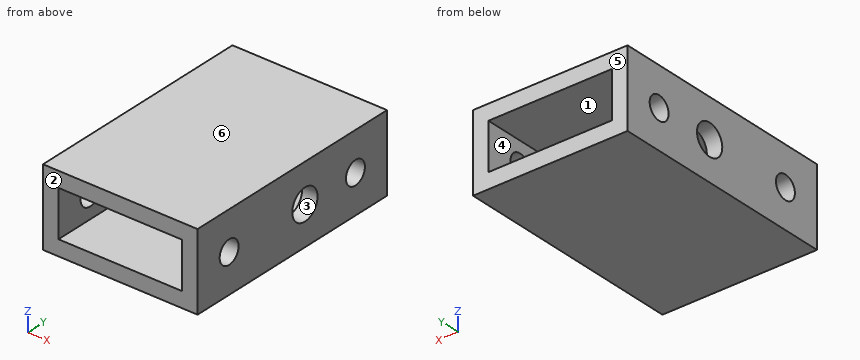
```python
from build123d import *

# Parameters (mm, degrees)
SKETCH_1_W          = 20
SKETCH_1_H          = 10
SKETCH_1_W_2        = 16
SKETCH_1_H_2        = 6
EXTRUDE_1_DEPTH     = 15
SKETCH_2_R          = 2
SKETCH_2_R_2        = 1.5
CUT_EXTRUDE_1_DEPTH = 26.495097568


with BuildPart() as part:
    # 草图1 → 凸台-拉伸1 (new, symmetric)
    with BuildSketch(Plane(origin=(0, 0, 0), x_dir=(1, 0, 0), z_dir=(0, 1, 0))):
        Rectangle(SKETCH_1_W, SKETCH_1_H)
        Rectangle(SKETCH_1_W_2, SKETCH_1_H_2, mode=Mode.SUBTRACT)
    extrude(amount=EXTRUDE_1_DEPTH, both=True)

    # 草图2 → 切除-拉伸1 (cut, through all)
    with BuildSketch(Plane.ZY.offset(10)):
        with Locations((0, 2)):
            Circle(SKETCH_2_R)
        with Locations((0, 10)):
            Circle(SKETCH_2_R_2)
        with Locations((0, -10)):
            Circle(SKETCH_2_R_2)
    extrude(amount=-CUT_EXTRUDE_1_DEPTH, mode=Mode.SUBTRACT)


solid = part.part
```
Geometry check sheet. Reference: the model listing, model coordinates, mm. Face numbers are marked on the shaded views. A direction names the side the tool comes from. Round coordinates to 2 decimals unless told otherwise and drop trailing zeros. Loops run counter-clockwise (first coordinate to the right, second up) from the corner with the lowest first, then second, coordinate; pieces in that order, holes last. Notation, with made-up numbers: (80.5, 28) - (108.5, 28) arc R9 ccw to (108.5, 43) - close; hole circle Ø9 at (25.5, 41.5). An arc over 180 degrees is marked (long way). Write each question's results on one line, items separated by ' | '. Start each with the question number.
Q1. Access from +Z, -Z, +X, -X, +Y, -Y to the whole of each face (thin tool, end or side, straight path). Record for the marked faces 1 and 2.
Q2. Thickness scan on line 1 (Y direction, x = 8.95, z = 0); line 2 (X direction, y = -3, z = -0.75); line 3 (Z direction, x = -3.75, y = -9.25). Record the ranges inside material, lowest first. Write a range as [from, to].
Q3. Cross-section at D-D on y = -4.25. Enter the section's corners in (x, z), and give its area (3 significant figures).
Q4. Cross-section at B-B on x = 1.5. Enter the section's corners in (y, z).
Q5. Gauge pin test, flat end, axial feed: P1, Ø2, axis at x = 1.5, z = 2.5, coming from the -Y side. Record the tip position at first contact, or that the pin passes through.
Q6. Cross-section at A-A on y = 10. Enter the section's corners in (x, z), and give its area (3 significant figures).
Q7. Release check for a two-part mould opening along Z. For the marked faces 3, 4, 5 and 6 record: +Z half, -Z half, draft (parallel to the pull), parting line (faces both ways), or undercut.
Q8. Cross-section at C-C on z = 0. State how many separate pieces and enclosed holes the cut face has, and give its area (3 significant figures).
Answers below:
1) face 1: +Y, -Y | face 2: +Z, -Z, +X, -X, -Y
2) line 1: y = [-15, -11.5], [-8.5, 0], [4, 8.5], [11.5, 15] | line 2: x = [-10, -8], [8, 10] | line 3: z = [-5, -3], [3, 5]
3) outline: (-10, -5) - (10, -5) - (10, 5) - (-10, 5) - close; hole (-8, -3) - (8, -3) - (8, 3) - (-8, 3) - close | area: 104 mm²
4) outline: (-15, -5) - (15, -5) - (15, -3) - (-15, -3) - close; (-15, 3) - (15, 3) - (15, 5) - (-15, 5) - close
5) P1: stops at y = -15
6) outline: (-10, -5) - (10, -5) - (10, -1.5) - (8, -1.5) - (8, -3) - (-8, -3) - (-8, -1.5) - (-10, -1.5) - close; (-10, 1.5) - (-8, 1.5) - (-8, 3) - (8, 3) - (8, 1.5) - (10, 1.5) - (10, 5) - (-10, 5) - close | area: 92.0 mm²
7) face 3: undercut | face 4: undercut | face 5: draft | face 6: +Z half
8) separate pieces: 8 | enclosed holes: 0 | area: 80.0 mm²
